Verification items for the finished model (mm, model axes). Round coordinates to 2 decimals unless told otherwise and drop trailing zeros. Write each loop counter-clockwise with the first axis right and the second up, starting at its lowest first coordinate (ties: lowest second). Pieces come first, ordered by that corner, then holes. Notation, with made-up numbers: (35.25, 53.5) - (54.25, 53.5) arc R18 cw to (54.25, 73.5) - close; hole circle Ø4 at (2.5, 75). An arc over 180 degrees is marked (long way). Answer as a JSON object with one key per item and string values. Group by question number.
1) Thickness scan on line 1 (Z direction, x = -0.5, y = 5.5); line 2 (Y direction, x = 1, z = 5.5); line 3 (Z direction, x = 4.5, y = -4.5). Record the ranges inside material, lowest first.
2) Section check A-A (z = 54.5). Enter the section's corners in (x, y) (3 decimals), then the cut area to 3 significant figures.
3) Go/stop test with flat-tipped pins: pin 1 Ø6 at (x, z) = (-2.5, 35.5) entering from -Y (3 decimals); pin 2 Ø3 at (y, z) = (-3.5, 51.5) entering from +X; pin 3 Ø6 at (y, z) = (-0.5, 14.5) entering from -X; pin 4 Ø5 at (x, z) = (-5.5, 56.5) entering from +Y. Record where each tip stops, or that it passes through.
```python
from build123d import *

# Parameters (mm, degrees)
F2_R     = 2.725
F3_DEPTH = 7.5
F4_R     = 2.725
F5_DEPTH = 7.5


with BuildPart() as f1:
    # F0 (on Front) → F1 (revolve)
    with BuildSketch(Plane.XZ):
        with BuildLine():
            Line((0, 70), (0, 3.15))
            Line((0, 3.15), (1, 3.15))
            add(Edge.make_bspline(
                [(1, 3.15), (2.04091373, 2.841939317), (4.1227411901, 2.2258179509), (5.7075803967, 0.741939317), (6.5, 0)],
                knots=[0, 0, 0, 0, 0.5, 1, 1, 1, 1], degree=3))
            Line((6.5, 0), (7.5, 0))
            Line((7.5, 0), (7.5, 3.15))
            add(Edge.make_bspline(
                [(7.5, 3.15), (5.2801080633, 6.8420764949), (3.0602161266, 10.5341529899), (2.675, 16.5)],
                knots=[0, 0, 0, 0, 0.3422357012, 0.3422357012, 0.3422357012, 0.3422357012], degree=3))
            add(Edge.make_bspline(
                [(2.675, 16.5), (2.5909368652, 17.8018868292), (2.5942435778, 19.2120538145), (2.675, 20.7182066219)],
                knots=[0.3422357012, 0.3422357012, 0.3422357012, 0.3422357012, 0.4169195057, 0.4169195057, 0.4169195057, 0.4169195057], degree=3))
            Line((2.675, 20.7182066219), (2.675, 63.65))
            Line((2.675, 63.65), (0.75, 70))
            Line((0.75, 70), (0, 70))
        make_face()
        with BuildLine():
            Line((2.675, 16.5), (2.675, 20.7182066219))
            add(Edge.make_bspline(
                [(2.675, 16.5), (2.5909368652, 17.8018868292), (2.5942435778, 19.2120538145), (2.675, 20.7182066219)],
                knots=[0.3422357012, 0.3422357012, 0.3422357012, 0.3422357012, 0.4169195057, 0.4169195057, 0.4169195057, 0.4169195057], degree=3))
        make_face()
    revolve(axis=Axis((0, 0, 35), (0, 0, 1)))

    # F2 (on Front) → F3 (cut, symmetric)
    with BuildSketch(Plane.XZ):
        Circle(F2_R)
    extrude(amount=F3_DEPTH, both=True, mode=Mode.SUBTRACT)

    # F4 (on Right) → F5 (cut, symmetric)
    with BuildSketch(Plane.YZ):
        Circle(F4_R)
    extrude(amount=F5_DEPTH, both=True, mode=Mode.SUBTRACT)


solid = f1.part
```
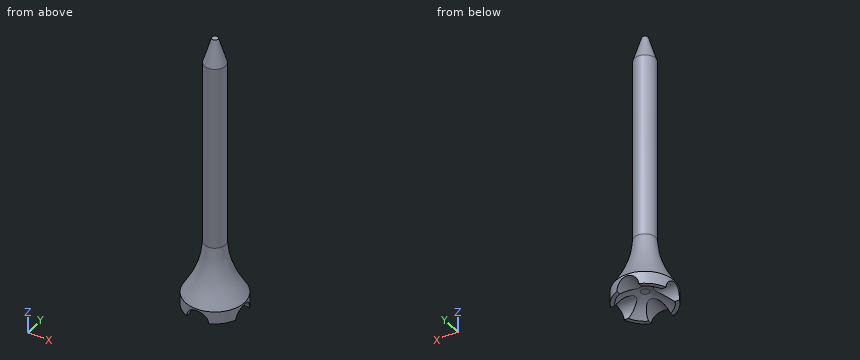
Returned:
{
 "1": {"line 1": "2.68 to 6.59", "line 2": "-6.03 to 6.03", "line 3": "0.13 to 5.07"},
 "2": {"outline": "circle Ø5.35 at (0, 0)", "area": "22.5 mm2"},
 "3": {"pin 1": "y = -2.675", "pin 2": "x = 1.78", "pin 3": "x = -3.51", "pin 4": "through"}
}
